Autodesk Inventor part; units mm, degrees
ref_plane "YZ Plane" through (0, 0, 0) normal (1, 0, 0) x (0, 1, 0)
ref_plane "XZ Plane" through (0, 0, 0) normal (0, 1, 0) x (-1, 0, 0)
ref_plane "XY Plane" through (0, 0, 0) normal (0, 0, 1) x (1, 0, 0)
sketch "Sketch1" plane through (0, 0, 0) normal (0, 0, 1) x (1, 0, 0)
  line L0 (0, 44) -> (44, 44) construction
  line L1 (44, 44) -> (44, 0) construction
  line L2 (44, 0) -> (0, 0) construction
  line L3 (0, 0) -> (0, 44) construction
  line L4 (3, 41) -> (41, 41) construction
  line L5 (41, 41) -> (41, 3) construction
  line L6 (41, 3) -> (3, 3) construction
  line L7 (3, 3) -> (3, 41) construction
  circle A0 centre (3, 41) radius 1.5
  circle A1 centre (41, 41) radius 1.5
  circle A2 centre (41, 3) radius 1.5
  circle A3 centre (3, 3) radius 1.5
  line L8 (44, 3) -> (44, 44) construction
  line L9 (48, 41) -> (86, 41) construction
  line L10 (86, 41) -> (86, 3) construction
  line L11 (86, 3) -> (48, 3) construction
  line L12 (48, 3) -> (48, 41) construction
  circle A4 centre (48, 41) radius 1.5
  circle A5 centre (48, 3) radius 1.5
  circle A6 centre (86, 3) radius 1.5
  circle A7 centre (86, 41) radius 1.5
  line L13 (45, 44) -> (89, 44) construction
  line L14 (89, 44) -> (89, 0) construction
  line L15 (89, 0) -> (45, 0) construction
  line L16 (45, 0) -> (45, 44) construction
  line L17 (90, 44) -> (134, 44) construction
  line L18 (134, 44) -> (134, 0) construction
  line L19 (134, 0) -> (90, 0) construction
  line L20 (90, 0) -> (90, 44) construction
  line L21 (93, 41) -> (131, 41) construction
  line L22 (131, 41) -> (131, 3) construction
  line L23 (131, 3) -> (93, 3) construction
  line L24 (93, 3) -> (93, 41) construction
  circle A8 centre (93, 41) radius 1.5
  circle A9 centre (131, 41) radius 1.5
  circle A10 centre (131, 3) radius 1.5
  circle A11 centre (93, 3) radius 1.5
  line L25 (0, 0) -> (134, 0)
  line L26 (134, 0) -> (134, 44)
  line L27 (0, 44) -> (0, 0)
  line L28 (0, 44) -> (134, 44)
  point P0 (0, 0)
  point P1 (22, 41)
  point P2 (41, 22)
  point P3 (44, 22)
  point P4 (22, 44)
  point P5 (67, 41)
  point P6 (67, 44)
  point P7 (86, 22)
  point P8 (89, 22)
  point P9 (112, 41)
  point P10 (112, 44)
  point P11 (131, 22)
  point P12 (134, 22)
  dimension "d9" = 44
  dimension "d10" = 44
  dimension "d11" = 38
  dimension "d12" = 38
  dimension "d17" = 3
  dimension "d18" = 3
  dimension "d19" = 3
  dimension "d20" = 3
  dimension "d33" = 38
  dimension "d34" = 38
  dimension "d35" = 3
  dimension "d36" = 3
  dimension "d37" = 3
  dimension "d38" = 3
  dimension "d39" = 44
  dimension "d40" = 44
  dimension "d41" = 1
  dimension "d42" = 44
  dimension "d43" = 44
  dimension "d44" = 38
  dimension "d45" = 38
  dimension "d46" = 1
  dimension "d47" = 3
  dimension "d48" = 3
  dimension "d49" = 3
  dimension "d50" = 3
extrude "Extrusion1" add sketch "Sketch1" along normal blind 3
sketch "Sketch2" plane through (0, 0, 3) normal (0, 0, 1) x (1, 0, 0)
  circle A0 centre (93, 3) radius 1.5
  circle A1 centre (131, 3) radius 1.5
  circle A2 centre (131, 41) radius 1.5
  circle A3 centre (93, 41) radius 1.5
  circle A4 centre (86, 41) radius 1.5
  circle A5 centre (86, 3) radius 1.5
  circle A6 centre (48, 3) radius 1.5
  circle A7 centre (48, 41) radius 1.5
  circle A8 centre (3, 3) radius 1.5
  circle A9 centre (41, 3) radius 1.5
  circle A10 centre (41, 41) radius 1.5
  circle A11 centre (3, 41) radius 1.5
  line L0 (0, 44) -> (0, 0) construction
  line L1 (0, 0) -> (134, 0) construction
  line L2 (134, 0) -> (134, 44) construction
  circle A12 centre (131, 41) radius 1.5
  circle A13 centre (131, 41) radius 3
  circle A14 centre (131, 3) radius 3
  circle A15 centre (93, 3) radius 3
  circle A16 centre (86, 3) radius 3
  circle A17 centre (48, 3) radius 3
  circle A18 centre (41, 3) radius 1.5
  circle A19 centre (41, 3) radius 3
  circle A20 centre (3, 3) radius 1.5
  circle A21 centre (3, 3) radius 3
  circle A22 centre (3, 41) radius 1.5
  circle A23 centre (3, 41) radius 3
  circle A24 centre (41, 41) radius 1.5
  circle A25 centre (41, 41) radius 3
  circle A26 centre (48, 41) radius 1.5
  circle A27 centre (48, 41) radius 3
  circle A28 centre (93, 41) radius 3
  circle A29 centre (86, 41) radius 3
  line L3 (134, 44) -> (0, 44)
  point P0 (0, 0)
  dimension "d70" = 6
  dimension "d71" = 6
  dimension "d72" = 6
  dimension "d73" = 6
  dimension "d74" = 6
  dimension "d75" = 6
  dimension "d76" = 6
  dimension "d77" = 6
  dimension "d79" = 6
  dimension "d80" = 6
  dimension "d83" = 6
  dimension "d84" = 6
extrude "Extrusion2" add sketch "Sketch2" along normal blind 3
sketch "Sketch8" plane through (0, 0, 3) normal (0, 0, 1) x (1, 0, 0)
  circle A0 centre (22, 22) radius 1.5
  circle A1 centre (112, 22) radius 1.5
  circle A2 centre (3, 41) radius 1.5 construction
  line L0 (3, 41) -> (3, 3) construction
  line L1 (3, 41) -> (41, 41) construction
  circle A3 centre (93, 41) radius 1.5 construction
  line L2 (93, 41) -> (131, 41) construction
  circle A4 centre (41, 41) radius 1.5 construction
  circle A5 centre (131, 41) radius 1.5 construction
  circle A6 centre (3, 3) radius 1.5 construction
  point P0 (0, 0)
  point P1 (3, 22)
  point P2 (112, 41)
  point P3 (22, 41)
  dimension "d117" = 3
  dimension "d118" = 3
extrude "Extrusion8" cut sketch "Sketch8" against normal through all
properties part number "BP003" material "ABS Plastic"
Verification items for the finished model (mm, model axes). A direction names the side the tool comes from. Give positions to 0.01 mm unless a question says otherwise; leave off trailing zeros. Write each loop counter-clockwise with the first axis right and the second up, starting at its lowest first coordinate (ties: lowest second). Pieces come first, ordered by that corner, then holes. Notation, with made-up numbers: (49.5, -2.5) - (61.5, -2.5) arc R26 ccw to (61.5, 30.5) - close; hole circle Ø8 at (-0.5, -11). An arc over 180 degrees is marked (long way). Put each result on its own line as item: value.
Q1. Section check C-C on z = 1.1. Count the separate pieces of the cut face and the enclosed holes in it, and give its area (3 significant figures).
Result:
separate pieces: 1
enclosed holes: 14
area: 5,800 mm2
Q2. Section check B-B on y = 22. Record the cut outline in (x, z).
Result:
outline: (0, 0) - (20.5, 0) - (20.5, 3) - (0, 3) - close; (23.5, 0) - (110.5, 0) - (110.5, 3) - (23.5, 3) - close; (113.5, 0) - (134, 0) - (134, 3) - (113.5, 3) - close
Q3. Section check D-D on x = 29.5. Record the cut outline in (y, z), and give its area (3 significant figures).
Result:
outline: (0, 0) - (44, 0) - (44, 3) - (0, 3) - close
area: 132 mm2
Q4. Set-up check for faces 4 (the face through (133.3, 43.4, 3)), 5 (the face through (0.6, 0.7, 3)), 6 (the face through (2.675, 42.464, 2.958)), 7 (the face through (66, 0, 1)), 8 (the face through (45.79, 38.97, 4.48)): record each of +Z, -Z, +X, -X, +Y, -Y from which the full face is reachable in a straight line by a thin tool's end or side.
Result:
face 4: +Z, +X, +Y
face 5: +Z, -X, -Y
face 6: +Z, -Z
face 7: +Z, -Z, +X, -X, -Y
face 8: +Z
Q5. Depth check by flat-ended pin: P1, Ø2.5, axis at x = 48, y = 3, coming from the +Z side; P2, Ø1, axis at x = 33.5, y = 34, coming from the +Z side. Enter the tip coordinate at first touch or a pass-through.
Result:
P1: through
P2: z = 3
Q6. Section check A-A on x = 112. Record the cut outline in (y, z).
Result:
outline: (0, 0) - (20.5, 0) - (20.5, 3) - (0, 3) - close; (23.5, 0) - (44, 0) - (44, 3) - (23.5, 3) - close
Q7. Scan lines: probe 1 along Y at (x, z) = (86, 1.7); probe 2 along Y at (x, z) = (112, 2.1); probe 3 along Z at (x, y) = (124, 4.5). Record each from-to range of solid material in increasing order. Write a range as from..to.
Result:
probe 1: 0..1.5, 4.5..39.5, 42.5..44
probe 2: 0..20.5, 23.5..44
probe 3: 0..3
Q8. Mould release check, pull along X, two halves, no side actions. Record for faces 1 (the face through (132.3, 39.7, 6)), 2 (the face through (0, 22, 1)), 3 (the face through (0.6, 4.8, 4.5)): released by +X, released by -X, zero draft, split by the parting line, or undercut.
Result:
face 1: zero draft
face 2: released by -X
face 3: undercut
